Could you check a few things on this drawing? It's one solid part, dimensions in mm from its lowest x, y, z. Give positions to 0.01 mm unless a question says otherwise; leave off trailing zeros. Order: outer loops, then holes, each group sorted by start corner. A loop starts at its lowest first (then second) coordinate and runs counter-clockwise, first axis right, second up. Notation, with made-up numbers: (-33, 32) - (16, 32) arc R27 cw to (16, 60) - close; hole circle Ø10 at (10, 85.5). An arc over 180 degrees is marked (long way). One line per question, with ' | ' between items. Start each with the question number.
1. Imagine slicing it at B-B (y = 0.8). Give the number of separate pieces and of enclosed holes in the cut face, and give its area (3 significant figures).
2. Imagine slicing it at C-C (x = 25.4). Please give me the cut outline in (y, z) (1 decimal), and give its area (3 significant figures).
3. Imagine slicing it at D-D (z = 40.5). Please give me the cut outline in (x, y) (3 decimals), and give its area (3 significant figures).
4. I need wall thicknesses on probe 1 along Z at (x, y) = (13, 2.1); probe 2 along X at (y, z) = (1.4, 37); probe 3 along Z at (x, y) = (25.4, 2.05). Which ranges of each line are inside material? Lowest first, please. Write a range as from..to.
5. For P1, Ø5.5, axis at x = 12.7, z = 38.1, coming from the +Y side; P2, Ø8.5, axis at x = 38.1, z = 38.1, coming from the +Y side (3 decimals); P3, Ø1, axis at y = 0.5, z = 12.5, coming from the +X side, each with a flat end and sliding along its axis, tell me the tip position at first contact or that it passes through.
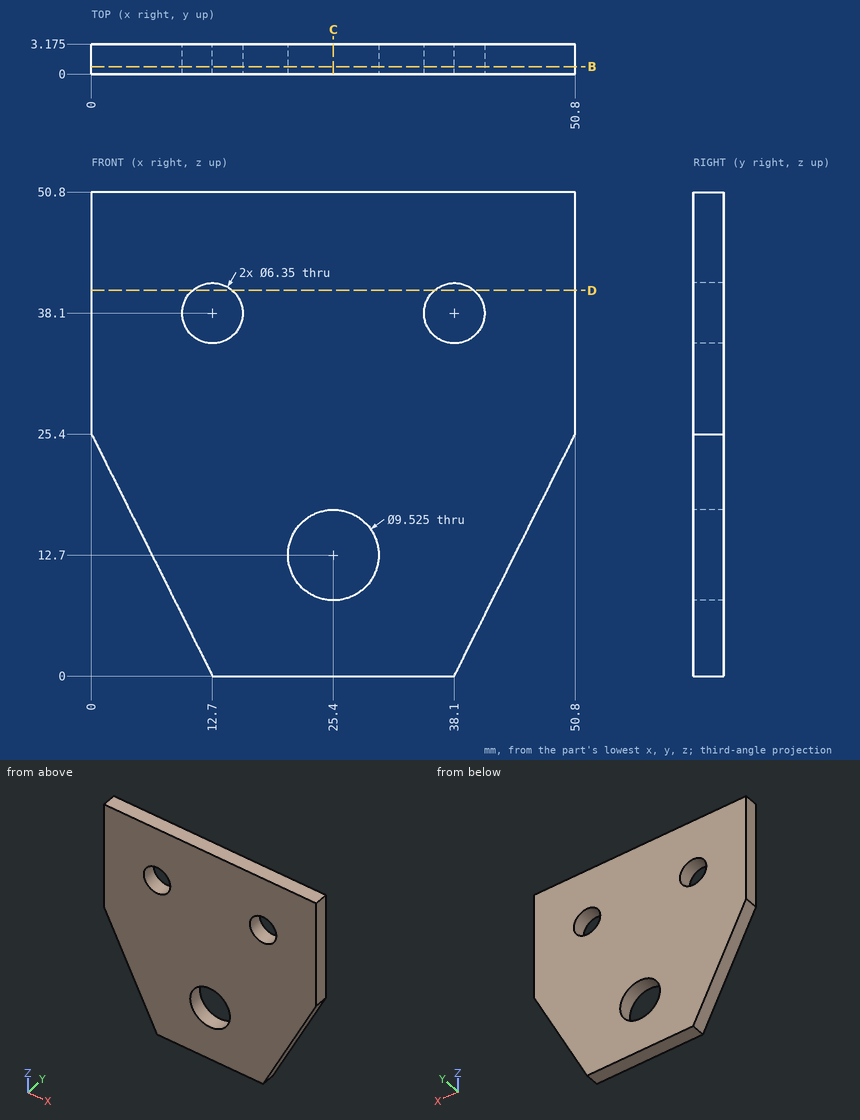
Results found:
1) separate pieces: 1 | enclosed holes: 3 | area: 2,120 mm2
2) outline: (0, 0) - (3.2, 0) - (3.2, 7.9) - (0, 7.9) - close; (0, 17.5) - (3.2, 17.5) - (3.2, 50.8) - (0, 50.8) - close | area: 131 mm2
3) outline: (0, 0) - (10.621, 0) - (10.621, 3.175) - (0, 3.175) - close; (14.779, 0) - (36.021, 0) - (36.021, 3.175) - (14.779, 3.175) - close; (40.179, 0) - (50.8, 0) - (50.8, 3.175) - (40.179, 3.175) - close | area: 135 mm2
4) probe 1: z = 0..34.94, 41.26..50.8 | probe 2: x = 0..9.72, 15.68..35.12, 41.08..50.8 | probe 3: z = 0..7.94, 17.46..50.8
5) P1: passes through | P2: stops at y = 3.175 | P3: stops at x = 44.6
